Input: dimensioned drawing with shaded views. Units: mm. Origin: part minimum x, y, z. Coordinates: 2 decimals unless noted, no trailing zeros. Order: outer loops, then holes, each group sorted by start corner. A loop starts at its lowest first (then second) coordinate and runs counter-clockwise, first axis right, second up. Notation, with made-up numbers: (17, 33) -> (32, 33) arc R23 ccw to (32, 67) -> close; hole circle Ø4 at (17, 21). An arc over 180 degrees is marked (long way). Put each result on its own line as item: value.
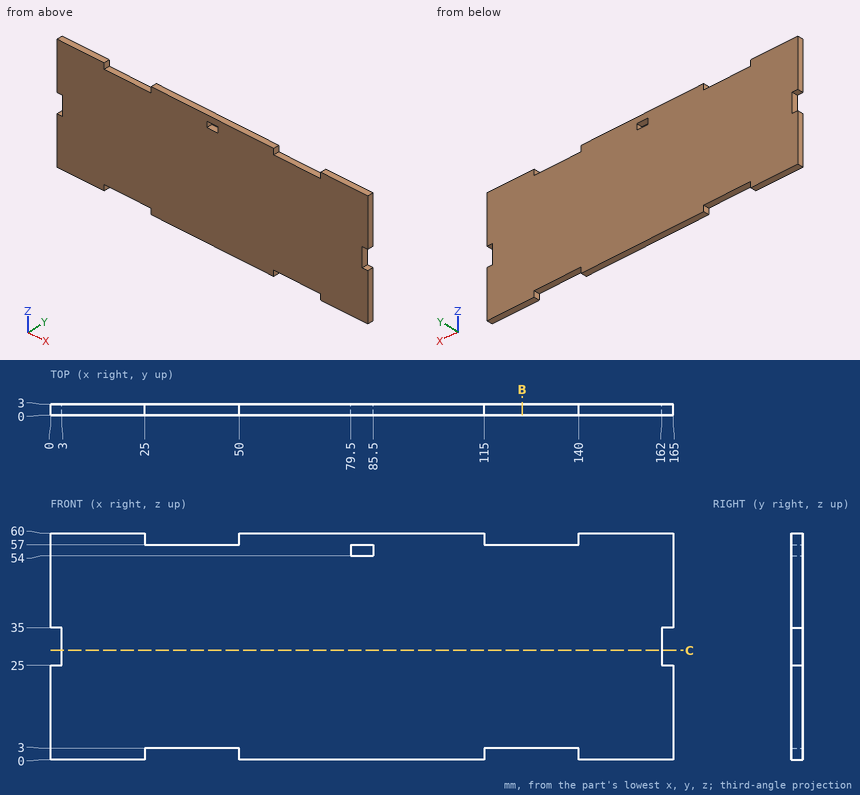
1. Cut plane B-B on x = 125. Output: boundary loops of the cut face in (y, z), plus the area to 3 significant figures.
Numbers:
outline: (0, 3) -> (3, 3) -> (3, 57) -> (0, 57) -> close
area: 162 mm2
2. First-contact query: pin 1 (0.9 mm diameter, centred on y = 1.5, z = 58, fed in from -X); pin 2 (0.9 mm diameter, centred on x = 38, y = 2, fed in from -Z); pin 3 (1.5 mm diameter, centred on x = 124, y = 1.5, fed in from +Z); pin 4 (0.9 mm diameter, centred on y = 2, z = 32, fed in from +X). Flat tips, straight axial feed; report the tip coordinate or a pass-through.
Numbers:
pin 1: stops at x = 0
pin 2: stops at z = 3
pin 3: stops at z = 57
pin 4: stops at x = 162
3. Ray query, line 1 along X through (y, z) = (1.05, 54.5); line 2 along Z through (x, y) = (127.5, 2.55); line 3 along X through (y, z) = (1, 31). Return the intervals inside material, ascending.
Numbers:
line 1: x = 0 to 79.5, 85.5 to 165
line 2: z = 3 to 57
line 3: x = 3 to 162
4. Cut plane C-C on z = 29. Output: boundary loops of the cut face in (x, y).
Numbers:
outline: (3, 0) -> (162, 0) -> (162, 3) -> (3, 3) -> close
